Part model, mm, in its own coordinate system. A direction names the side the tool comes from. Give positions to 0.01 mm unless a question says otherwise; leave off trailing zeros. Write each loop counter-clockwise with the first axis right and the second up, starting at its lowest first coordinate (ties: lowest second). Pieces come first, ordered by that corner, then holes.
from build123d import *

# Parameters (mm, degrees)
SKETCH1_W           = 21.5
SKETCH1_H           = 44
BOSS_EXTRUDE2_DEPTH = 3
SKETCH1_8_W         = 10
SKETCH1_8_H         = 20
CUT_EXTRUDE1_DEPTH  = 1.5
BOSS_EXTRUDE3_DEPTH = 45.25
SKETCH2_W           = 10
SKETCH2_H           = 10
BOSS_EXTRUDE4_DEPTH = 3
CHAMFER4_SIZE       = 5.25


with BuildPart() as part:
    # Sketch1 → Boss-Extrude2 (new body)
    with BuildSketch(Plane(origin=(0, 0, 0), x_dir=(1, 0, 0), z_dir=(0, 1, 0))):
        with Locations((-10.75, 22)):
            Rectangle(SKETCH1_W, SKETCH1_H)
    extrude(amount=BOSS_EXTRUDE2_DEPTH)

    # Sketch1<8> → Cut-Extrude1 (cut)
    with BuildSketch(Plane(origin=(0, 0, 0), x_dir=(1, 0, 0), z_dir=(0, 1, 0))):
        with Locations((-5, 22)):
            Rectangle(SKETCH1_8_W, SKETCH1_8_H)
    extrude(amount=CUT_EXTRUDE1_DEPTH, mode=Mode.SUBTRACT)

    # Sketch1<9> → Boss-Extrude3 (add)
    with BuildSketch(Plane(origin=(0, 0, 0), x_dir=(1, 0, 0), z_dir=(0, 1, 0))):
        Polygon((-21.5, 0), (-21.5, 7), (-24.5, 7), (-24.5, -3), (-14.5, -3), (-14.5, 0), align=None)
        Polygon((-24.5, 37), (-21.5, 37), (-21.5, 44), (-14.5, 44), (-14.5, 47), (-24.5, 47), align=None)
    extrude(amount=BOSS_EXTRUDE3_DEPTH)

    # Sketch2 → Boss-Extrude4 (add)
    with BuildSketch(Plane(origin=(0, 45.25, 0), x_dir=(1, 0, 0), z_dir=(0, 1, 0))):
        with Locations((-19.5, 2)):
            Rectangle(SKETCH2_W, SKETCH2_H)
        with Locations((-19.5, 42)):
            Rectangle(SKETCH2_W, SKETCH2_H)
    extrude(amount=BOSS_EXTRUDE4_DEPTH)

    # Chamfer4
    chamfer4_edges = [part.edges().sort_by_distance(p)[0] for p in [
        (-21.5, 24.125, 0),
        (-21.5, 24.125, -44),
    ]]
    chamfer(chamfer4_edges, length=CHAMFER4_SIZE)


solid = part.part
1) Saw through at B-B (x = -15.25). Write the cut outline in (y, z).
Check result:
outline: (0, -47) - (48.25, -47) - (48.25, -37) - (45.25, -37) - (45.25, -44) - (3, -44) - (3, 0) - (45.25, 0) - (45.25, -7) - (48.25, -7) - (48.25, 3) - (0, 3) - close
2) Saw through at A-A (y = 23.5). Write the cut outline in (x, z).
Check result:
outline: (-24.5, -47) - (-14.5, -47) - (-14.5, -44) - (-16.25, -44) - (-21.5, -38.75) - (-21.5, -37) - (-24.5, -37) - close; (-24.5, -7) - (-21.5, -7) - (-21.5, -5.25) - (-16.25, 0) - (-14.5, 0) - (-14.5, 3) - (-24.5, 3) - close
3) Saw through at C-C (x = -23). Write the cut outline in (y, z), and give its area (3 significant figures).
Check result:
outline: (0, -47) - (48.25, -47) - (48.25, -37) - (0, -37) - close; (0, -7) - (48.25, -7) - (48.25, 3) - (0, 3) - close
area: 965 mm2
4) Mould opens along Y. For faces 4 (the flat face through (-20, 48.25, -2)), 5 (the flat face through (-21.5, 1, -22)), 6 (the flat face through (-18.91, 23.83, -41.34)) say: +Y half, -Y half, draft (parallel to the pull), parting line (faces both ways), or undercut.
Check result:
face 4: +Y half
face 5: draft
face 6: undercut
5) Flat gauge pins, fed straight in: P1, Ø1.9, axis at y = 20, z = -38, coming from the +X side; P2, Ø1.5, axis at x = -8, y = 1.5, coming from the +Z side; P3, Ø1.9, axis at y = 17.5, z = -6.5, coming from the +X side; P4, Ø3, axis at y = 5.5, z = -21, coming from the -X side. Where does each tip first touch, or does it go through?
Check result:
P1: stops at x = -21.3
P2: stops at z = 0
P3: stops at x = -21.5
P4: passes through
6) Saw through at D-D (z = -20.5). Write the cut outline in (x, y).
Check result:
outline: (-21.5, 0) - (-10, 0) - (-10, 1.5) - (0, 1.5) - (0, 3) - (-21.5, 3) - close
7) 3-axis set-ups, long thin cutter, end or side, ignore diameter. For faces 1 (the flat face through (-5, 1, -32)), 2 (the flat face through (-17, 45.25, -4)), 3 (the flat face through (-7, 1, -44)): which of +Z, -Z, +X, -X, +Y, -Y reach the whole face in a straight line?
Check result:
face 1: +X, -Y
face 2: +X
face 3: -Z, +X, +Y, -Y
8) Drill centre lines: L1, parallel to Y at x = -21, z = -30; L2, parallel to Z at x = -20, y = 44.5; L3, parallel to Z at x = -16.5, y = 35.5. Where is each one in solid material? Low to high.
Check result:
L1: y = 0 to 3
L2: z = -47 to -40.25, -3.75 to 3
L3: z = -47 to -43.75, -0.25 to 3
